from build123d import *

# Parameters (mm, degrees)
SKETCH1_R           = 2
BOSS_EXTRUDE1_DEPTH = 30
BOSS_EXTRUDE2_DEPTH = 2


with BuildPart() as part:
    # Sketch1 → Boss-Extrude1 (new body)
    with BuildSketch(Plane(origin=(0, 0, 0), x_dir=(1, 0, 0), z_dir=(0, 1, 0))):
        with Locations((76.558114335, 38.393702022)):
            Circle(SKETCH1_R)
    extrude(amount=BOSS_EXTRUDE1_DEPTH)

    # Sketch2 → Boss-Extrude2 (add)
    with BuildSketch(Plane.XZ):
        Polygon((79.569925871, -34.594742746), (73.5463028, -34.594742746), (69.687221965, -41.602416762), (83.429006706, -41.602416762), align=None)
    extrude(amount=BOSS_EXTRUDE2_DEPTH)


solid = part.part
Can you work these out from the model? Positions are in its coordinate system, mm. A direction names the side the tool comes from. Give positions to 0.01 mm unless a question says otherwise; leave off trailing zeros. Loops run counter-clockwise (first coordinate to the right, second up) from the corner with the lowest first, then second, coordinate; pieces in that order, holes last. Notation, with made-up numbers: M 69.25,-8 L 113.25,-8 A14 cw 113.25,17 Z; hole C -10.5,17 d1. An arc over 180 degrees is marked long. One line per item, written item: value. Start each with the question number.
1) If we section it at D-D, the plane x = 81.75: Write out the boundary of the cut face in (y, z).
2) If we section it at A-A, the plane x = 75.25: Write out the boundary of the cut face in (y, z), and give its area (3 significant figures).
3) If we section it at B-B, the plane z = -37.25: Write out the boundary of the cut face in (x, y), and give its area (3 significant figures).
4) If we section it at C-C, the plane y = 15: Write out the boundary of the cut face in (x, z), and give its area (3 significant figures).
5) I'm going to push flat-ended pins straight in: pin 1 (1.5 mm diameter, centred on x = 71.5, z = -39.5, fed in from +Y); pin 2 (4 mm diameter, centred on y = 14, z = -37, fed in from -X); pin 3 (3 mm diameter, centred on y = 19.5, z = -35.5, fed in from -X). Where does each tip first touch, or does it pass through?
6) On a 3-axis mill with a long thin cutter (end or side, diameter ignored), from which of +Z, -Z, +X, -X, +Y, -Y can I reach the whole of each face in a straight line? I mean faces 1 (the face through (76, -1, -41.602)), 2 (the face through (75, 0, -40)). Say none if no direction works.
7) If I drill on line 1 (Y direction, x = 80, z = -41); line 2 (X direction, y = 9, z = -39.75); line 3 (X direction, y = 16.5, z = -37.5), over which ranges is the centre line in solid material (lowest first)? Write a range as [from, to].
Completed:
1. outline: M -2,-41.6 L 0,-41.6 L 0,-38.55 L -2,-38.55 Z
2. outline: M -2,-41.6 L 0,-41.6 L 0,-39.91 L 30,-39.91 L 30,-36.88 L 0,-36.88 L 0,-34.59 L -2,-34.59 Z
2. area: 105 mm^2
3. outline: M 72.08,-2 L 81.03,-2 L 81.03,0 L 78.2,0 L 78.2,30 L 74.92,30 L 74.92,0 L 72.08,0 Z
3. area: 116 mm^2
4. outline: C 76.56,-38.39 d4
4. area: 12.6 mm^2
5. pin 1: stops at y = 0
5. pin 2: stops at x = 74.56
5. pin 3: stops at x = 75.12
6. face 1: -Z, +X, -X, +Y, -Y
6. face 2: +Y
7. line 1: y = [-2, 0]
7. line 2: x = [75.09, 78.03]
7. line 3: x = [74.77, 78.35]
